Source: CAD feature listing. Evaluate the final solid. Frame: model axes, mm. A direction names the side the tool comes from. Give positions to 0.01 mm unless a question says otherwise; leave off trailing zeros. Order: outer loops, then holes, each group sorted by start corner. A loop starts at its lowest first (then second) coordinate and runs counter-clockwise, first axis right, second up. Notation, with made-up numbers: (2.5, -13) -> (35.5, -13) arc R32 cw to (35.5, 20) -> close; hole circle Ø6 at (-16.75, 86.5). An arc over 180 degrees is marked (long way). Use CSV: the item, a comma, the result in double quotes.
```python
from build123d import *

# Parameters (mm, degrees)
BOSS_EXTRUDE1_DEPTH = 10
BOSS_EXTRUDE2_DEPTH = 30
SKETCH3_W           = 5
SKETCH3_H           = 25
BOSS_EXTRUDE3_DEPTH = 22.5
SKETCH4_R           = 5.25
CUT_EXTRUDE1_DEPTH  = 27
SKETCH5_R           = 2.7
CUT_EXTRUDE3_DEPTH  = 4.6
CUT_EXTRUDE4_DEPTH  = 44.5
CUT_EXTRUDE5_REACH  = 67.133
FILLET1_R           = 4
FILLET2_R           = 0.5
FILLET3_R           = 5
FILLET4_R           = 0.5


with BuildPart() as part:
    # Sketch1 → Boss-Extrude1 (new body)
    with BuildSketch(Plane.XY):
        with BuildLine():
            Line((-22.5, 15.75), (-28.5, 9.75))
            Line((-28.5, 9.75), (-28.5, 9.25))
            Line((-28.5, 9.25), (-28.5, 1.75))
            Line((-28.5, 1.75), (-17.5, -9.25))
            Line((-17.5, -9.25), (28.5, -9.25))
            Line((28.5, -9.25), (28.5, 9.25))
            Line((28.5, 9.25), (0.8, 9.25))
            Line((0.8, 9.25), (-3.5, 13.55))
            Line((-3.5, 13.55), (-3.5, 9.25))
            Line((-3.5, 9.25), (-13.382383367, 9.25))
            ThreePointArc((-13.382383367, 9.25), (-23.330458604, 1.863270054), (-13.985855563, 10))
            Line((-13.985855563, 10), (-4.25, 10))
            Line((-4.25, 10), (-4.25, 14.3))
            Line((-4.25, 14.3), (-5.7, 15.75))
            Line((-5.7, 15.75), (-22.5, 15.75))
        make_face()
    extrude(amount=BOSS_EXTRUDE1_DEPTH)

    # Sketch2 → Boss-Extrude2 (add)
    with BuildSketch(Plane(origin=(28.5, 0, 0), x_dir=(0, 0, -1), z_dir=(1, 0, 0))):
        Polygon((-10, 9.25), (-10, -9.25), (-26.933078921, -15.75), (-32, -15.75), (-32, 9.25), align=None)
    extrude(amount=-BOSS_EXTRUDE2_DEPTH)

    # Sketch3 → Boss-Extrude3 (add)
    with BuildSketch(Plane.XY.offset(32)):
        with Locations((1, -3.25)):
            Rectangle(SKETCH3_W, SKETCH3_H)
    extrude(amount=BOSS_EXTRUDE3_DEPTH)

    # Sketch4 → Cut-Extrude1 (cut)
    with BuildSketch(Plane(origin=(0, 0, 0), x_dir=(-1, 0, 0), z_dir=(0, 0, -1))):
        with Locations((-18.5, -0.75)):
            Circle(SKETCH4_R)
    extrude(amount=-CUT_EXTRUDE1_DEPTH, mode=Mode.SUBTRACT)

    # Sketch5 → Cut-Extrude3 (cut)
    with BuildSketch(Plane.XY.offset(32)):
        with Locations((18.5, -0.75)):
            Circle(SKETCH5_R)
    extrude(amount=-CUT_EXTRUDE3_DEPTH, mode=Mode.SUBTRACT)

    # Sketch6 → Cut-Extrude4 (cut)
    with BuildSketch(Plane.XY.offset(54.5)):
        Polygon((-1.5, 9.25), (2, 9.25), (-1.5, 3.25), align=None)
    extrude(amount=-CUT_EXTRUDE4_DEPTH, mode=Mode.SUBTRACT)

    # Sketch7 → Cut-Extrude5 (cut, up to next)
    with BuildSketch(Plane(origin=(3.5, 0, 0), x_dir=(0, 0, -1), z_dir=(1, 0, 0)), mode=Mode.PRIVATE) as cut_extrude5_sk1:
        with BuildLine():
            Line((-47, -5.95), (-54.5, -5.95))
            Line((-54.5, -5.95), (-54.5, -0.55))
            Line((-54.5, -0.55), (-47, -0.55))
            ThreePointArc((-47, -0.55), (-44.3, -3.25), (-47, -5.95))
        make_face()
    cut_extrude5_tool1 = extrude(cut_extrude5_sk1.sketch, amount=-CUT_EXTRUDE5_REACH, mode=Mode.PRIVATE) & part.part
    add(cut_extrude5_tool1.solids().sort_by_distance((3.5, -3.25, 49.670838))[0], mode=Mode.SUBTRACT)

    # Fillet1
    fillet1_edges = [part.edges().sort_by_distance(p)[0] for p in [
        (-17.5, -9.25, 5),
        (-28.5, 1.75, 5),
        (-28.5, 9.75, 5),
        (-22.5, 15.75, 5),
    ]]
    fillet(fillet1_edges, radius=FILLET1_R)

    # Fillet2
    fillet2_edges = [part.edges().sort_by_distance(p)[0] for p in [
        (3.5, -15.75, 43.25),
        (3.5, 9.25, 43.25),
        (-1.5, 3.25, 32.25),
        (2, 9.25, 32.25),
        (-13.985855563, 10, 5),
        (-13.382383367, 9.25, 5),
        (-3.5, 13.55, 5),
        (-4.25, 14.3, 5),
        (28.5, 9.25, 16),
        (0.8, 9.25, 5),
        (-5.7, 15.75, 5),
    ]]
    fillet(fillet2_edges, radius=FILLET2_R)

    # Fillet3
    fillet3_edges = [part.edges().sort_by_distance(p)[0] for p in [
        (13.5, -9.25, 10),
        (13.5, -15.75, 26.933078921),
    ]]
    fillet(fillet3_edges, radius=FILLET3_R)

    # Fillet4
    # the kernel refuses this fillet: 0.5 mm, written as the material it takes off along each edge
    with BuildSketch(Plane(origin=(28.5, -15.75, 27.859774145), x_dir=(-1, 0, 0), z_dir=(0, 0, 1))) as fillet4_piece_1:
        with BuildLine():
            CenterArc((FILLET4_R, -FILLET4_R), FILLET4_R, 90, 90)
            Line((0, -FILLET4_R), (0, 0))
            Line((0, 0), (FILLET4_R, 0))
        make_face()
    extrude(amount=5.390225855, mode=Mode.SUBTRACT)
    with BuildSketch(Plane(origin=(28.5, -10.75, 27.859774145), x_dir=(0, -1, 0), z_dir=(0, 0, 1))) as fillet4_piece_2:
        with BuildLine():
            CenterArc((5 - FILLET4_R, -FILLET4_R), FILLET4_R, 0, 90)
            Line((5, -FILLET4_R), (5, 0))
            Line((5, 0), (5 - FILLET4_R, 0))
        make_face()
    revolve(axis=Axis((28.5, -10.75, 27.859774145), (1, 0, 0)), revolution_arc=21, mode=Mode.SUBTRACT)
    with BuildSketch(Plane(origin=(28.5, -9.25, -1.25), x_dir=(0, 1, 0), z_dir=(0, 0, 1))) as fillet4_piece_3:
        with BuildLine():
            CenterArc((FILLET4_R, FILLET4_R), FILLET4_R, 180, 90)
            Line((0, FILLET4_R), (0, 0))
            Line((0, 0), (FILLET4_R, 0))
        make_face()
    extrude(amount=10.323304775, mode=Mode.SUBTRACT)
    with BuildSketch(Plane(origin=(28.5, -14.25, 9.073304775), x_dir=(0, 0.9335804264972017, 0.35836794954530055), z_dir=(0, -0.35836794954530055, 0.9335804264972017))) as fillet4_piece_4:
        with BuildLine():
            CenterArc((5 + FILLET4_R, FILLET4_R), FILLET4_R, 180, 90)
            Line((5, FILLET4_R), (5, 0))
            Line((5, 0), (5 + FILLET4_R, 0))
        make_face()
    revolve(axis=Axis((28.5, -14.25, 9.073304775), (-1, 0, 0)), revolution_arc=21, mode=Mode.SUBTRACT)
    with BuildSketch(Plane(origin=(-1.5, -14.25, 9.073304775), x_dir=(0, 0.9335804264972017, 0.35836794954530055), z_dir=(0, -0.35836794954530055, 0.9335804264972017))) as fillet4_piece_5_section:
        with BuildLine():
            CenterArc((5 + FILLET4_R, -FILLET4_R), FILLET4_R, 90, 90)
            Line((5, -FILLET4_R), (5, 0))
            Line((5, 0), (5 + FILLET4_R, 0))
        make_face()
    fillet4_piece_5 = revolve(axis=Axis((-1.5, -14.25, 9.073304775), (-1, 0, 0)), revolution_arc=35.324258071, mode=Mode.PRIVATE)
    fillet4_piece_5 = split(fillet4_piece_5, bisect_by=Plane(origin=(-1.457320012, -9.164080053, 10), z_dir=(0, 0, 1)), keep=Keep.TOP, mode=Mode.PRIVATE)
    add(fillet4_piece_5, mode=Mode.SUBTRACT)
    with BuildSketch(Plane(origin=(-1.5, -14.25, 9.073304775), x_dir=(0, 0.9335804264972017, 0.35836794954530055), z_dir=(0, -0.35836794954530055, 0.9335804264972017))) as fillet4_piece_6_section:
        with BuildLine():
            CenterArc((5 + FILLET4_R, -FILLET4_R), FILLET4_R, 90, 90)
            Line((5, -FILLET4_R), (5, 0))
            Line((5, 0), (5 + FILLET4_R, 0))
        make_face()
    fillet4_piece_6 = revolve(axis=Axis((-1.5, -14.25, 9.073304775), (-1, 0, 0)), revolution_arc=35.324258071, mode=Mode.PRIVATE)
    fillet4_piece_6 = split(fillet4_piece_6, bisect_by=Plane(origin=(-1.316288707, -9.25, 9.750524402), z_dir=(0, -1, 0)), keep=Keep.TOP, mode=Mode.PRIVATE)
    add(fillet4_piece_6, mode=Mode.SUBTRACT)
    with BuildSketch(Plane(origin=(-1.5, -9.582097868, 10.865144523), x_dir=(0, 0.9335804264972015, 0.3583679495453009), z_dir=(0, -0.3583679495453009, 0.9335804264972015))) as fillet4_piece_7:
        with BuildLine():
            CenterArc((FILLET4_R, -FILLET4_R), FILLET4_R, 90, 90)
            Line((0, -FILLET4_R), (0, 0))
            Line((0, 0), (FILLET4_R, 0))
        make_face()
    extrude(amount=16.284392263, mode=Mode.SUBTRACT)
    with BuildSketch(Plane(origin=(28.5, -9.582097868, 10.865144523), x_dir=(0, 0.9335804264972015, 0.3583679495453009), z_dir=(0, -0.3583679495453009, 0.9335804264972015))) as fillet4_piece_8:
        with BuildLine():
            CenterArc((FILLET4_R, FILLET4_R), FILLET4_R, 180, 90)
            Line((0, FILLET4_R), (0, 0))
            Line((0, 0), (FILLET4_R, 0))
        make_face()
    extrude(amount=16.284392263, mode=Mode.SUBTRACT)
    with BuildSketch(Plane(origin=(-1.5, -10.75, 27.859774145), x_dir=(0, -1, 0), z_dir=(0, 0, 1))) as fillet4_piece_9:
        with BuildLine():
            CenterArc((5 - FILLET4_R, FILLET4_R), FILLET4_R, 270, 90)
            Line((5 - FILLET4_R, 0), (5, 0))
            Line((5, 0), (5, FILLET4_R))
        make_face()
    revolve(axis=Axis((-1.5, -10.75, 27.859774145), (1, 0, 0)), revolution_arc=21, mode=Mode.SUBTRACT)
    with BuildSketch(Plane(origin=(-1.5, -15.75, 27.859774145), x_dir=(1, 0, 0), z_dir=(0, 0, 1))) as fillet4_piece_10:
        with BuildLine():
            CenterArc((FILLET4_R, FILLET4_R), FILLET4_R, 180, 90)
            Line((0, FILLET4_R), (0, 0))
            Line((0, 0), (FILLET4_R, 0))
        make_face()
    extrude(amount=27.890225855, mode=Mode.SUBTRACT)

    # Sketch8 → Cut-Revolve1 (revolve, cut)
    with BuildSketch(Plane.XY.offset(5), mode=Mode.PRIVATE) as cut_revolve1_sk:
        Polygon((-8.5, 15.75), (-6.75, 15.75), (-6.75, -4.25), (-6.15, -4.25), (-6.15, -8.75), (-6, -8.75), (-6, -9.25), (-8.5, -9.25), align=None)
    revolve(cut_revolve1_sk.sketch.rotate(Axis((-8.5, 24.852937644, 5), (0, -1, 0)), 180), axis=Axis((-8.5, 24.852937644, 5), (0, -1, 0)), mode=Mode.SUBTRACT)


with BuildPart() as body_2:
    # Mirror1: mirrored copy
    add(part.part.mirror(Plane(origin=(0, 0, 0), x_dir=(0, 0, 1), z_dir=(1, 0, 0))))


solid = body_2.part
```
1. Section query A-A on x = 8.5. Return loops of the section in (y, z), plus the area to 3 significant figures.
Answer below:
outline,"(-9.25, 0) -> (9.25, 0) -> (9.25, 3.25) -> (-4.25, 3.25) -> (-4.25, 2.65) -> (-8.75, 2.65) -> (-8.75, 2.5) -> (-9.25, 2.5) -> close; (-9.25, 7.5) -> (-8.75, 7.5) -> (-8.75, 7.35) -> (-4.25, 7.35) -> (-4.25, 6.75) -> (9.25, 6.75) -> (9.25, 10) -> (-9.25, 10) -> close; (10, 0) -> (15.75, 0) -> (15.75, 3.25) -> (10, 3.25) -> close; (10, 6.75) -> (15.75, 6.75) -> (15.75, 10) -> (10, 10) -> close"
area,"151 mm²"
2. Mould query, pull axis Y, two halves, no side actions, for faces 5 (the cylindrical face through (22.354, 15.454, 5.07)), 6 (the flat face through (-1, -5.95, 51)), 7 (the flat face through (-28.5, 0, 16)). Classes: released by +Y, released by -Y, zero draft, split by the parting line, or undercut.
Answer below:
face 5,"released by +Y"
face 6,"undercut"
face 7,"zero draft"
3. Ray query, line 1 along Y through (x, z) = (-18.5, 28.95); line 2 along X through (y, z) = (1.5, 5); line 3 along X through (y, z) = (-1.5, 5). Return the intervals inside material, ascending.
Answer below:
line 1,"y = -15.75 to -3.45, 1.95 to 9.25"
line 2,"x = -28.5 to -23.24, -13.76 to 6.75, 10.25 to 13.99, 23.01 to 28.02"
line 3,"x = -28.5 to -23.7, -13.3 to 6.75, 10.25 to 25.25"
4. Access query for faces 1 (the cylindrical face through (-23.745, -0.519, 13.311)), 2 (the cylindrical face through (-21.075, 0.061, 29.732)), 3 (the flat face through (-1, -0.55, 51)), 4 (the cylindrical face through (10.885, -9.004, 4.249)). Directions: +Z, -Z, +X, -X, +Y, -Y. A direction counts if a zero-diameter tool reaches every point of the face in a straight line with its end or side. Return the directions, or none.
Answer below:
face 1,"-Z"
face 2,"+Z"
face 3,"+Z, +X, -X"
face 4,"-Y"
5. Section query C-C on y = 6. Return loops of the section in (x, z).
Answer below:
outline,"(-28.5, 0) -> (12.31, 0) -> (12.31, 10) -> (-0.1, 10) -> (-0.1, 54.5) -> (-3.5, 54.5) -> (-3.5, 32) -> (-28.5, 32) -> close; (24.69, 0) -> (28.5, 0) -> (28.5, 10) -> (24.69, 10) -> close; hole circle Ø3.5 at (8.5, 5)"
6. Pin query (flat end, axial travel): P1, Ø3, axis at x = 18, z = 6.5, coming from the -Y side; P2, Ø6.5, axis at x = -18.5, y = -0.75, coming from the +Z side; P3, Ø5.5, axis at y = -4, z = 33.5, coming from the +X side; P4, Ø3, axis at x = 8.5, z = 5, coming from the -Y side. Return the tip coordinate at first contact, or that it passes through.
Answer below:
P1,"stops at y = -9.2"
P2,"stops at z = 32"
P3,"stops at x = 1.5"
P4,"passes through"
7. Section query B-B on z = 48.5. Return loops of the section in (x, y), plus the area to 3 significant figures.
Answer below:
outline,"(-3.5, -15.25) arc R0.5 ccw to (-3, -15.75) -> (1, -15.75) arc R0.5 ccw to (1.5, -15.25) -> (1.5, -5.95) -> (-3.5, -5.95) -> close; (-3.5, -0.55) -> (1.5, -0.55) -> (1.5, 3.11) arc R0.5 ccw to (1.43, 3.37) -> (-1.86, 9) arc R0.5 ccw to (-2.29, 9.25) -> (-3, 9.25) arc R0.5 ccw to (-3.5, 8.75) -> close"
area,"87.3 mm²"
8. Section query D-D on x = -18.5. Return loops of the section in (y, z).
Answer below:
outline,"(-15.75, 27.86) arc R5 ccw to (-15.42, 26.07) -> (-9.58, 10.87) arc R5 cw to (-9.25, 9.07) -> (-9.25, 0) -> (-6, 0) -> (-6, 27) -> (4.5, 27) -> (4.5, 0) -> (9.25, 0) -> (9.25, 32) -> (1.95, 32) -> (1.95, 27.4) -> (-3.45, 27.4) -> (-3.45, 32) -> (-15.75, 32) -> close"
